The model under review builds one solid part; all positions refer to its coordinate system, in mm. A direction names the side the tool comes from. Coordinates: 2 decimals unless noted, no trailing zeros. Loops run counter-clockwise (first coordinate to the right, second up) from the corner with the lowest first, then second, coordinate; pieces in that order, holes last. Notation, with made-up numbers: M 75.5,21.25 L 82.5,21.25 A8 cw 82.5,26.25 Z; hole C -5,53 d1. An arc over 180 degrees is marked long. Use CSV: the item, a comma, the result in double quotes. Start each with the question number.
1. Clearance check with flat-ended pins moving along their axes: P1, Ø0.6, axis at x = 4, z = 4, coming from the -Y side; P2, Ø2, axis at x = 1.5, z = 1, coming from the -Y side; P3, Ø1, axis at x = -10, z = -2.5, coming from the -Y side. State where each tip first meets the part, or that it passes through.
2. Draft analysis for pull direction X (two halves, no side actions). For faces 1 (the flat face through (1, 0, 0)), 2 (the cylindrical face through (-1.1, 1.8, 0.5)), 3 (the cylindrical face through (-7.02, -0.45, -2.87)), state which applies: +X half, -X half, draft (parallel to the pull), parting line (faces both ways), or undercut.
3. Add section B-B, the plane x = 5. Write out the cut boundary in (y, z).
4. For L1, parallel to Y at x = 7, z = -0.25; L2, parallel to X at y = -0.6, z = 1; L3, parallel to X at y = 1.7, z = 0, list the stretches that pass through material, from the lowest coordinate up.
5. Add section C-C, the plane y = 2.1. Write out the cut boundary in (x, z).
6. Tool access review of faces 4 (the flat face through (-12, -1.194, 0)), 5 (the flat face through (5, 1.016, 4)), 6 (the flat face through (-3.8, -0.4, 3.366)), 7 (the cylindrical face through (-6.514, 0.515, 0.405)), 8 (the flat face through (-12.573, 1, 0)): name each direction out of +Z, -Z, +X, -X, +Y, -Y from which nothing blocks a thin tool from reaching the whole face with its end or side.
7. Add section A-A, the plane z = 0. Write out the cut boundary in (x, y).
8. Add section D-D, the plane x = -10. Write out the cut boundary in (y, z), then the cut area to 3 significant figures.
Autodesk Inventor part; units mm, degrees
ref_plane "YZ Plane" through (0, 0, 0) normal (1, 0, 0) x (0, 1, 0)
ref_plane "XZ Plane" through (0, 0, 0) normal (0, 1, 0) x (-1, 0, 0)
ref_plane "XY Plane" through (0, 0, 0) normal (0, 0, 1) x (1, 0, 0)
sketch "Sketch1" plane through (0, 0, 0) normal (1, 0, 0) x (0, 1, 0)
  line L0 (-2.1432, 0) -> (4.5023, 0)
  line L1 (0, 7.0231) -> (0, -7.0231)
  line L2 (2.54, -5.0165) -> (2.54, 5.0165)
  line L3 (2.54, 5.0165) -> (0, 5.0165)
  line L4 (0, 5.0165) -> (0, -5.0165)
  line L5 (0, -5.0165) -> (2.54, -5.0165)
  line L6 (2.54, -5.0165) -> (0, 5.0165) construction
  line L7 (2.54, 5.0165) -> (0, -5.0165) construction
  line L8 (0, 3.0734) -> (1.016, 3.0734)
  line L9 (1.016, 3.0734) -> (1.016, 5.0165)
  line L10 (0, -3.0734) -> (1.016, -3.0734)
  line L11 (1.016, -3.0734) -> (1.016, -5.0165)
  line L12 (1.27, 0) -> (3.553, 0) construction
  point P0 (0, 0)
  dimension "d0" = 10.033
  dimension "d1" = 2.54
  dimension "d2" = 0
  dimension "d3" = 1.016
  dimension "d4" = 6.1468
  dimension "d5" = 1.9431
  dimension "d6" = 1.9431
extrude "Extrusion1" add sketch "Sketch1" along normal blind 9.906 contours L1 L8 L9 L3 L2 L0 | L0 L2 L5 L11 L10 L1
extrude "Extrusion2" add sketch "Sketch1" against normal blind 12.573
sketch "Sketch2" plane through (0, 0, 0) normal (0, 1, 0) x (-1, 0, 0)
  line L0 (-2.3558, 0) -> (14.1351, 0)
  line L1 (0, -4.445) -> (0, 4.445)
  point P0 (0, 0)
  point P1 (3.429, 0)
  dimension "d11" = 3.429
hole "Hole1" at (-3.429, 0, 0) direction (0, 1, 0) diameter 4.7625 end through all counterbore diameter 6.223 counterbore depth 1.016
sketch "Sketch3" plane through (9.906, 0, -3.0734) normal (0, -1, 0) x (1, 0, 0)
  line L0 (-22.479, 6.4389) -> (-17.399, 6.4389)
  line L1 (-17.399, 6.4389) -> (-17.399, -0.2921)
  line L2 (-17.399, -0.2921) -> (-22.479, -0.2921)
  line L3 (-22.479, -0.2921) -> (-22.479, 6.4389)
  line L4 (-34.3558, 3.0734) -> (5.726, 3.0734)
  line L5 (-9.906, 10.1016) -> (-9.906, -3.9802)
  line L6 (-9.906, 3.0734) -> (-28.6298, 3.0734) construction
  line L7 (-22.479, 8.0899) -> (0, 8.0899)
  line L8 (-22.479, 6.4389) -> (-11.684, 6.4389)
  line L9 (-11.684, 6.4389) -> (-11.684, 8.0899)
  line L10 (-11.684, 8.0899) -> (-22.479, 8.0899)
  line L11 (-22.479, 8.0899) -> (-22.479, 6.4389)
  line L12 (0, -1.9431) -> (-22.479, -1.9431)
  line L13 (-22.479, -0.2921) -> (-11.684, -0.2921)
  line L14 (-11.684, -0.2921) -> (-11.684, -1.9431)
  line L15 (-11.684, -1.9431) -> (-22.479, -1.9431)
  line L16 (-22.479, -1.9431) -> (-22.479, -0.2921)
  dimension "d22" = 5.08
  dimension "d30" = 6.731
  dimension "d45" = 10.795
  dimension "d46" = 10.795
extrude "Extrusion3" add sketch "Sketch3" along normal blind 0.889 contours L11 L7 L9 L8 L0 | L0 L1 L4 L3 | L4 L1 L2 L3 | L2 L13 L14 L12 L16
chamfer "Chamfer2" distance 0.254 angle 45 2 edges at (-1.778, -0.889, 4.191) (-1.778, -0.889, -4.191)
fillet "Fillet1" radius 0.7937 2 edges at (9.906, 1.778, 5.0165) (9.906, 1.778, -5.0165)
fillet "Fillet2" [suppressed]
sketch "Sketch4" plane through (0, 0, 0) normal (0, 1, 0) x (-1, 0, 0)
  circle A0 centre (3.429, 0) radius 2.3813
  circle A1 centre (3.429, 0) radius 3.175
  point P0 (0, 0)
  dimension "d34" = 6.35
sketch "Sketch5" plane through (9.906, -0.889, -3.0734) normal (0, -1, 0) x (1, 0, 0)
  line L0 (-26.9748, 3.0734) -> (4.4958, 3.0734)
  line L1 (-9.906, 10.0965) -> (-9.906, -3.9497)
  line L2 (-22.479, 8.0899) -> (-22.479, -1.9431)
  line L3 (-20.955, -0.4191) -> (-22.479, -0.4191)
  line L4 (-22.479, -0.4191) -> (-22.479, 6.5659)
  line L5 (-22.479, 6.5659) -> (-20.955, 6.5659)
  line L6 (-20.955, 6.5659) -> (-20.955, -0.4191)
  line L7 (-20.955, -0.4191) -> (-22.479, 6.5659) construction
  line L8 (-22.479, -0.4191) -> (-20.955, 6.5659) construction
  point P0 (-9.906, 3.0734)
  point P1 (-21.717, 3.0734)
  dimension "d47" = 6.985
  dimension "d48" = 1.524
extrude "Extrusion4" add sketch "Sketch5" along normal blind 0.3048
chamfer "Chamfer4" distance 1.27 distance2 1.27 1 edges at (-12.573, 0.8255, -5.0165) measured on face at (-12.573, 1.397, 1.1642)
chamfer "Chamfer5" distance 1.27 distance2 1.27 1 edges at (-12.573, 0.8255, 5.0165) measured on face at (-9.0593, 0.254, 5.0165)
fillet "Fillet4" radius 0.7937 2 edges at (-12.573, -1.0414, -3.4925) (-12.573, -1.0414, 3.4925)
fillet "Fillet5" radius 0.7937 4 edges at (-12.573, 0.8255, 3.7465) (-11.303, 0.8255, 5.0165) (-12.573, 0.8255, -3.7465) (-11.303, 0.8255, -5.0165)
fillet "Fillet6" radius 1.651 4 edges at (0, 0.508, -3.0734) (0, 0.508, 3.0734) (-7.493, -0.4445, 3.3655) (-7.493, -0.4445, -3.3655)
sketch "Sketch6" plane through (0, 0, 0) normal (0, 0, 1) x (1, 0, 0)
  line L0 (-11.049, -1.1938) -> (-11.7793, -1.1938)
  line L1 (-11.049, -0.889) -> (-11.049, -1.1938)
  line L2 (-2.032, -0.889) -> (-10.9742, -0.889)
  line L3 (-11.049, -1.1938) -> (-2.032, -0.889)
  point P0 (0, 0)
  dimension "d51" = 1.936
chamfer "Chamfer6" distance 0.9652 angle 45 4 edges at (5.7785, 0, -3.0734) (0, 0, -4.8704) (5.7785, 0, 3.0734) (0, 0, 4.8704) measured on face at (7.1543, 0, 1.0245)
chamfer "Chamfer7" distance 0.9652 angle 45 1 edges at (9.906, 0, 0)
properties part number "J010513" material "STAINLESS STEEL, 303"
Computed:
1,P1,"stops at y = 1.02"
1,P2,"stops at y = 0"
1,P3,"stops at y = -0.89"
2,face 1,"draft"
2,face 2,"undercut"
2,face 3,"+X half"
3,outline,"M 0,-2.11 L 0.97,-3.07 L 1.02,-3.07 L 1.02,-5.02 L 2.54,-5.02 L 2.54,5.02 L 1.02,5.02 L 1.02,3.07 L 0.97,3.07 L 0,2.11 Z"
4,L1,"y = 0 to 2.54"
4,L2,"x = -12.57 to -7.49"
4,L3,"x = -12.57 to -5.81, -1.05 to 9.91"
5,outline,"M -12.57,-3.42 A0.79 ccw -12.34,-3.98 L -11.54,-4.78 A0.79 ccw -10.97,-5.02 L 9.11,-5.02 A0.79 ccw 9.91,-4.22 L 9.91,4.22 A0.79 ccw 9.11,5.02 L -10.97,5.02 A0.79 ccw -11.54,4.78 L -12.34,3.98 A0.79 ccw -12.57,3.42 Z; hole C -3.43,0 d4.76"
6,face 4,"+Z, -Z, +X, -X, -Y"
6,face 5,"+Z, +X, -Y"
6,face 6,"+X, -Y"
6,face 7,"-Y"
6,face 8,"+Z, -Z, -X, +Y, -Y"
7,outline,"M -12.57,-1.19 L -11.05,-1.19 L -11.05,-0.89 L -7.49,-0.89 L -7.49,0 L -6.54,0 L -6.54,1.02 L -5.81,1.02 L -5.81,2.54 L -12.57,2.54 Z; M -1.05,1.02 L -0.32,1.02 L -0.32,0 L 8.94,0 L 9.91,0.97 L 9.91,2.54 L -1.05,2.54 Z"
8,outline,"M -0.89,-5.02 L 2.54,-5.02 L 2.54,5.02 L -0.89,5.02 Z"
8,area,"34.4 mm^2"
